Here's how the part is built. I have some questions about the finished solid (model axes, mm). Face numbers are marked on the shaded views. A direction names the side the tool comes from. Coordinates: 2 decimals unless noted, no trailing zeros. Write each loop counter-clockwise with the first axis right and the second up, starting at its lowest first coordinate (ties: lowest second). Pieces come first, ordered by that corner, then holes. Notation, with made-up numbers: (34, -24.5) -> (65, -24.5) arc R12 ccw to (65, -2.5) -> close; hole circle Ø11 at (36, -40). An arc over 180 degrees is marked (long way). Use a Markdown table: item, result. Add a question column.
Item 1: On a 3-axis mill with a long thin cutter (end or side, diameter ignored), from which of +Z, -Z, +X, -X, +Y, -Y can I reach the whole of each face in a straight line? I mean the marked faces 1 and 2. Say none if no direction works.
Item 2: Imagine slicing it at D-D, the plane y = 5.35. Write out the boundary of the cut face in (x, z), and give its area (3 significant figures).
Item 3: Imagine slicing it at C-C, the plane z = -0.25. Write out the boundary of the cut face in (x, y), and give its area (3 significant figures).
Item 4: Imagine slicing it at A-A, the plane y = 4.7. Write out the boundary of the cut face in (x, z), and give its area (4 significant figures).
Item 5: Will this pin go through, and if not, where does the flat tip stop? pin 1 Ø1.5 at (x, y) = (-1, 4) entering from +Z.
Item 6: If I drill on line 1 along Z through (x, y) = (-1.45, 4.15); line 2 along X through (y, z) = (3.35, 0.8); line 3 along X through (y, z) = (0.5, 1.6), over which ranges is the centre line in solid material (lowest first)? Write a range as from..to.
Item 7: Imagine slicing it at B-B, the plane x = -2.1. Write out the boundary of the cut face in (y, z), and give its area (4 significant figures).
```python
from build123d import *

# Parameters (mm, degrees)
SKETCH1_W           = 6
SKETCH1_H           = 5
BOSS_EXTRUDE1_DEPTH = 6
CUT_EXTRUDE1_DEPTH  = 3.5
SKETCH3_W           = 3
SKETCH3_H           = 2
BOSS_EXTRUDE2_DEPTH = 3


with BuildPart() as part:
    # Sketch1 → Boss-Extrude1 (new body)
    with BuildSketch(Plane(origin=(0, 0, 0), x_dir=(1, 0, 0), z_dir=(0, 1, 0))):
        Rectangle(SKETCH1_W, SKETCH1_H)
    extrude(amount=BOSS_EXTRUDE1_DEPTH)

    # Sketch2 → Cut-Extrude1 (cut)
    with BuildSketch(Plane.XY.offset(2.5)):
        Polygon((3, 6), (-3, 0), (-3, 6), align=None)
    extrude(amount=-CUT_EXTRUDE1_DEPTH, mode=Mode.SUBTRACT)

    # Sketch3 → Boss-Extrude2 (add)
    with BuildSketch(Plane(origin=(0, 6, 0), x_dir=(1, 0, 0), z_dir=(0, 1, 0))):
        with Locations((1.5, 0)):
            Rectangle(SKETCH3_W, SKETCH3_H)
    extrude(amount=-BOSS_EXTRUDE2_DEPTH)


solid = part.part
```
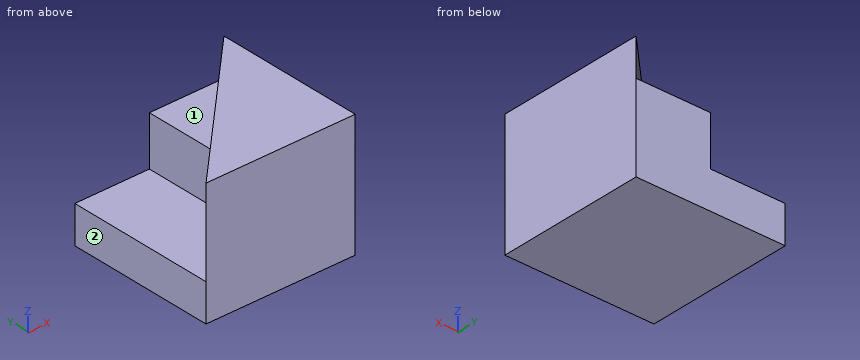
Ans:
| question | item | result |
|---|---|---|
| 1 | face 1 | +Z, -X, +Y |
| 1 | face 2 | +Z, -Z, -X, +Y, -Y |
| 2 | outline | (-3, -2.5) -> (3, -2.5) -> (3, 2.5) -> (2.35, 2.5) -> (2.35, 1) -> (0, 1) -> (0, -1) -> (-3, -1) -> close |
| 2 | area | 16.0 mm^2 |
| 3 | outline | (-3, 0) -> (3, 0) -> (3, 6) -> (0, 6) -> (0, 3) -> close |
| 3 | area | 22.5 mm^2 |
| 4 | outline | (-3, -2.5) -> (3, -2.5) -> (3, 2.5) -> (1.7, 2.5) -> (1.7, 1) -> (0, 1) -> (0, -1) -> (-3, -1) -> close |
| 4 | area | 16.95 mm^2 |
| 5 | pin 1 | stops at z = -1 |
| 6 | line 1 | z = -2.5..-1 |
| 6 | line 2 | x = 0..3 |
| 6 | line 3 | x = -2.5..3 |
| 7 | outline | (0, -2.5) -> (6, -2.5) -> (6, -1) -> (0.9, -1) -> (0.9, 2.5) -> (0, 2.5) -> close |
| 7 | area | 12.15 mm^2 |
